Could you check a few things on this drawing? It's one solid part, dimensions in mm from its lowest x, y, z. Give positions to 0.01 mm unless a question says otherwise; leave off trailing zeros. Order: outer loops, then holes, each group sorted by start corner. A loop starts at its lowest first (then second) coordinate and runs counter-clockwise, first axis right, second up. Notation, with made-up numbers: (-27, 49.5) - (17, 49.5) arc R36 cw to (17, 85.5) - close; hole circle Ø10 at (31.5, 68). An arc over 180 degrees is marked (long way). Answer as CSV lines item,"result".
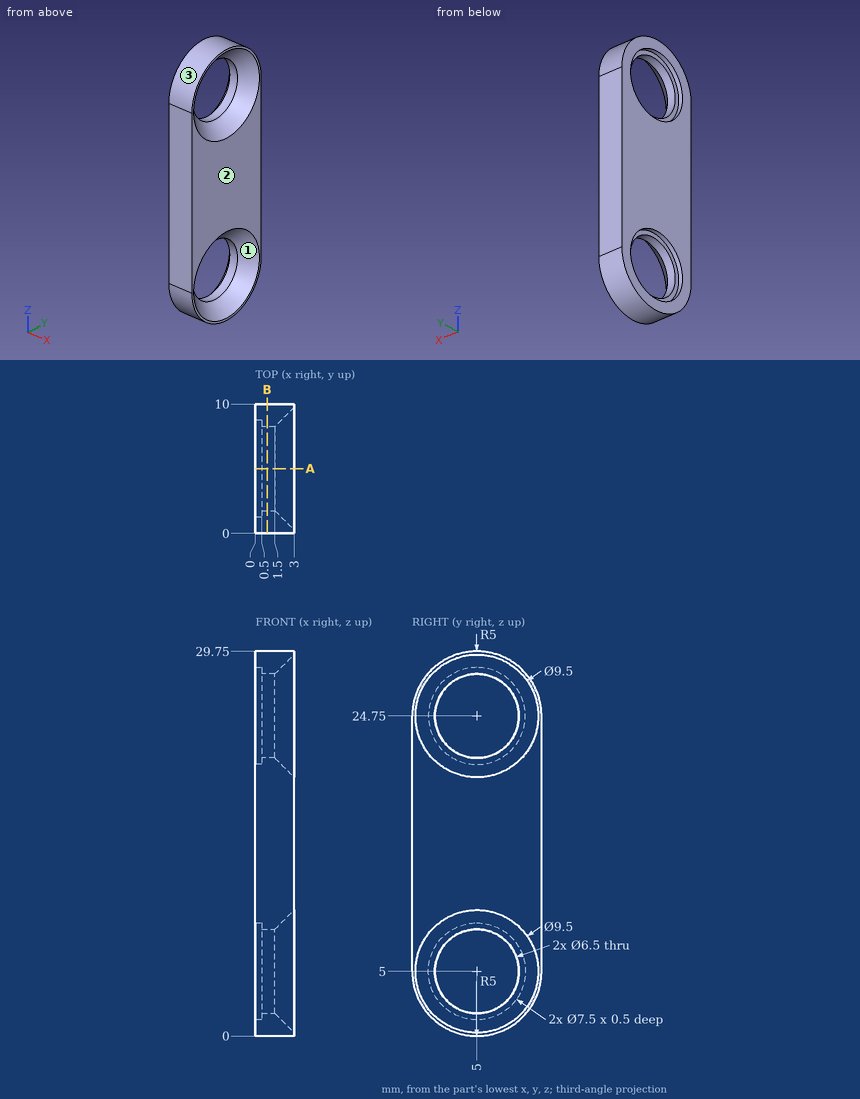
1) If we mould it in two halves opening along Y, with no side actions, what happens to the marked faces 1, 2 and 3? For each: +Y half, -Y half, draft (parallel to the pull), parting line (faces both ways), or undercut.
Answer block:
face 1,"undercut"
face 2,"draft"
face 3,"parting line"
2) I need wall thicknesses on line 1 along Z through (x, y) = (0.8, 5); line 2 along Y through (x, z) = (0.2, 24.75); line 3 along Z through (x, y) = (0.2, 6). Which ranges of each line are inside material? Lowest first, please. Write a range as [from, to].
Answer block:
line 1,"[0, 1.75], [8.25, 21.5], [28, 29.75]"
line 2,"[0, 1.25], [8.75, 10]"
line 3,"[0.1, 1.39], [8.61, 21.14], [28.36, 29.65]"
3) I'm going to push flat-ended pins straight in: P1, Ø1, axis at y = 6.5, z = 23.5, coming from the +X side; P2, Ø1.5, axis at x = 0.5, y = 3.5, coming from the -Z side. Where does each tip first touch, or does it pass through?
Answer block:
P1,"through"
P2,"z = 0.06"
4) I want a section at A-A on y = 5. Write out the boundary of the cut face in (x, z).
Answer block:
outline,"(0, 0) - (3, 0) - (3, 0.25) - (1.5, 1.75) - (0.5, 1.75) - (0.5, 1.25) - (0, 1.25) - close; (0, 8.75) - (0.5, 8.75) - (0.5, 8.25) - (1.5, 8.25) - (3, 9.75) - (3, 20) - (1.5, 21.5) - (0.5, 21.5) - (0.5, 21) - (0, 21) - close; (0, 28.5) - (0.5, 28.5) - (0.5, 28) - (1.5, 28) - (3, 29.5) - (3, 29.75) - (0, 29.75) - close"
5) I want a section at B-B on x = 0.9. Write out the boundary of the cut face in (y, z).
Answer block:
outline,"(0, 5) arc R5 ccw to (10, 5) - (10, 24.75) arc R5 ccw to (0, 24.75) - close; hole circle Ø6.5 at (5, 5); hole circle Ø6.5 at (5, 24.75)"
